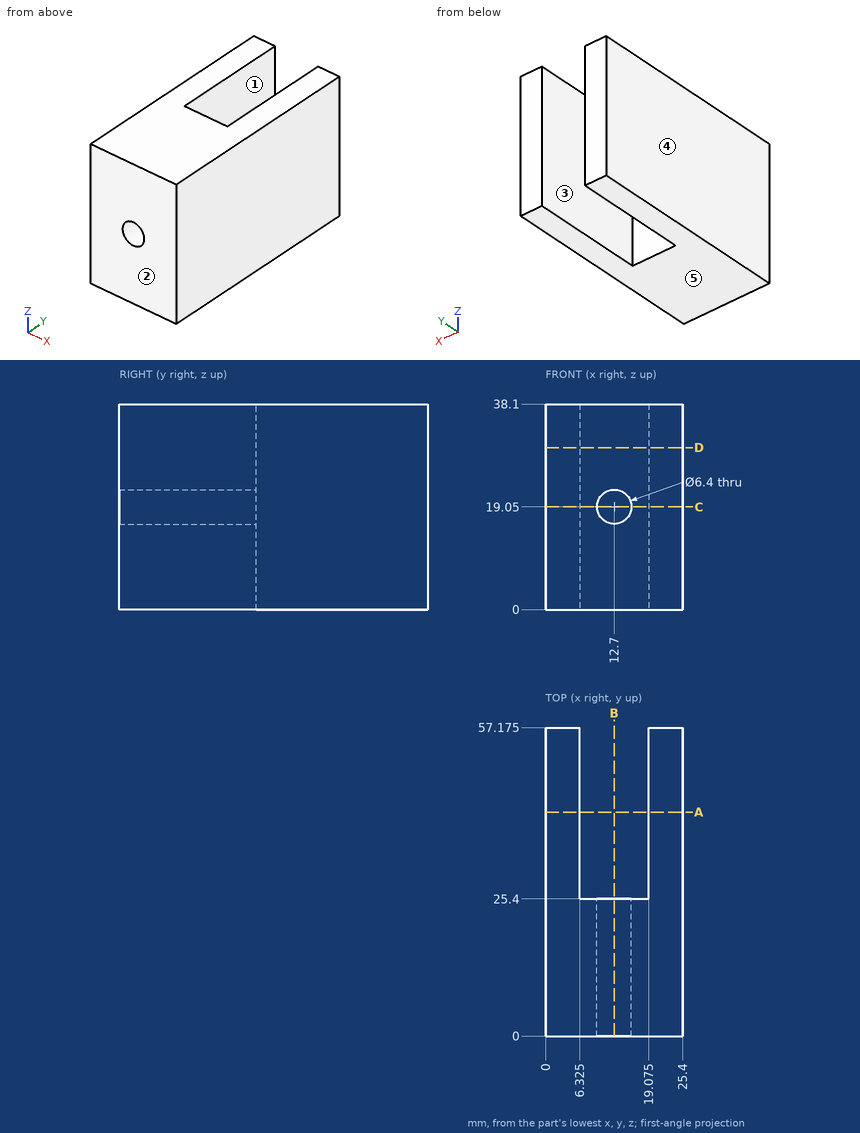
Check sheet for the drawn part. Datum: minimum x, y, z corner. Units: mm. A direction names the side the tool comes from. Round coordinates to 2 decimals unless told otherwise and drop trailing zeros. Order: outer loops, then holes, each group sorted by start corner. A loop starts at its lowest first (then second) coordinate and runs counter-clockwise, first axis right, second up. Notation, with made-up numbers: (22, -20) -> (77, -20) arc R27 ccw to (77, 11) -> close; hole circle Ø2 at (17.5, 2). An arc over 180 degrees is marked (long way). Use CSV: the item, a comma, the result in double quotes.
(1) Material ranges on line 1 along X through (y, z) = (51, 30) (3 decimals); line 2 along X through (y, z) = (8, 19); line 3 along Z through (x, y) = (12.7, 18.25), recorded low to high. Write a range as from..to.
Worked out:
line 1,"0..6.325, 19.075..25.4"
line 2,"0..9.5, 15.9..25.4"
line 3,"0..15.85, 22.25..38.1"
(2) Cross-section at A-A (y = 41.5). Record the boundary of the cut face in (x, z) (3 decimals).
Worked out:
outline,"(0, 0) -> (6.325, 0) -> (6.325, 38.1) -> (0, 38.1) -> close; (19.075, 0) -> (25.4, 0) -> (25.4, 38.1) -> (19.075, 38.1) -> close"
(3) Cross-section at D-D (z = 30). Record the boundary of the cut face in (x, y) (3 decimals), and give its area (3 significant figures).
Worked out:
outline,"(0, 0) -> (25.4, 0) -> (25.4, 57.175) -> (19.075, 57.175) -> (19.075, 25.4) -> (6.325, 25.4) -> (6.325, 57.175) -> (0, 57.175) -> close"
area,"1,050 mm²"
(4) Depth check by flat-ended pin: pin 1 (8.5 mm diameter, centred on x = 12.7, z = 19.05, fed in from -Y). Enter the tip coordinate at first touch or a pass-through.
Worked out:
pin 1,"y = 0"
(5) Tool access check on the marked faces 1 and 2. Record the directions out of +Z, -Z, +X, -X, +Y, -Y that give a thin tool (end or side, any length) a straight path to the whole face; none if there is none.
Worked out:
face 1,"+Z, -Z, +Y"
face 2,"+Z, -Z, +X, -X, -Y"
(6) Draft check along X on the marked faces 3, 4 and 5. Enter one of: pulls with the +X half, pulls with the -X half, needs draft (parallel to the pull), parting line crosses it, or undercut.
Worked out:
face 3,"undercut"
face 4,"pulls with the -X half"
face 5,"needs draft"
(7) Cross-section at C-C (z = 19.05). Record the boundary of the cut face in (x, y) (3 decimals).
Worked out:
outline,"(0, 0) -> (9.5, 0) -> (9.5, 25.4) -> (6.325, 25.4) -> (6.325, 57.175) -> (0, 57.175) -> close; (15.9, 0) -> (25.4, 0) -> (25.4, 57.175) -> (19.075, 57.175) -> (19.075, 25.4) -> (15.9, 25.4) -> close"
(8) Cross-section at B-B (x = 12.7). Record the boundary of the cut face in (y, z).
Worked out:
outline,"(0, 0) -> (25.4, 0) -> (25.4, 15.85) -> (0, 15.85) -> close; (0, 22.25) -> (25.4, 22.25) -> (25.4, 38.1) -> (0, 38.1) -> close"
